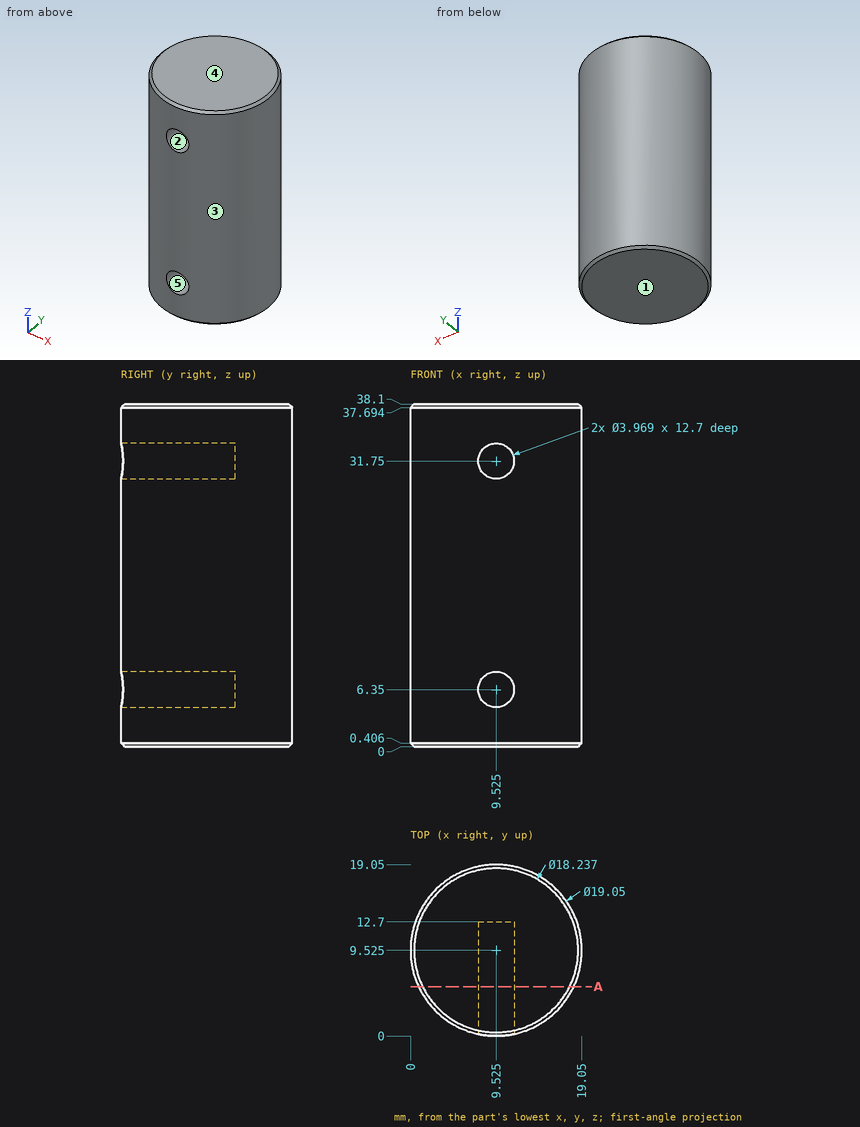
Geometry check sheet. Reference: drawing and pictorial views, mm from the part's lowest x, y, z. A direction names the side the tool comes from. Round coordinates to 2 decimals unless told otherwise and drop trailing zeros. One line per item, written item: value. Start each with the question number.
1. Gauge pin test, flat ends, axial feed: P1, Ø1.5, axis at y = 11, z = 24.5, coming from the +X side; P2, Ø4.5, axis at x = 10.5, z = 7, coming from the -Y side; P3, Ø3, axis at y = 4, z = 32.5, coming from the -X side; P4, Ø6, axis at x = 4, z = 25, coming from the +Y side. Record the tip position at first contact, or that the pin passes through.
2. Section check A-A on y = 5.5. Give the number of separate pieces and of enclosed holes in the cut face, and give its area (3 significant figures).
3. Access from +Z, -Z, +X, -X, +Y, -Y to the whole of each face (thin tool, end or side, straight path). Record for the marked faces 4 and 5.
4. Scan lines: line 1 along Z through (x, y) = (9.5, 4.25) (1 decimal); line 2 along Z through (x, y) = (8.5, 8.5); line 3 along X through (y, z) = (6.75, 6.35). Record each from-to range of solid material in increasing order.
5. Release check for a two-part mould opening along X. For the marked faces 1, 2 and 3 record: released by +X, released by -X, zero draft, split by the parting line, or undercut.
Results found:
1. P1: x = 19.02
1. P2: y = 0
1. P3: x = 0.89
1. P4: y = 18.71
2. separate pieces: 1
2. enclosed holes: 2
2. area: 633 mm^2
3. face 4: +Z, +X, -X, +Y, -Y
3. face 5: -Y
4. line 1: 0 to 4.4, 8.3 to 29.8, 33.7 to 38.1
4. line 2: 0 to 4.65, 8.05 to 30.05, 33.45 to 38.1
4. line 3: 0.41 to 7.54, 11.51 to 18.64
5. face 1: zero draft
5. face 2: undercut
5. face 3: split by the parting line
